from build123d import *

# Parameters (mm, degrees)
SKETCH10_W              = 71
SKETCH10_H              = 34
BOSS_EXTRUDE6_DEPTH     = 3.5
SKETCH11_R              = 1.55
CUT_EXTRUDE6_DEPTH      = 3.5
SKETCH12_R              = 2.75
CUT_EXTRUDE7_DEPTH      = 3.5
SKETCH13_R              = 3.75
BOSS_EXTRUDE7_DEPTH     = 25
CUT_EXTRUDE8_DEPTH      = 108.597630085
CUT_EXTRUDE8_DEPTH_BACK = 108.597630085
SKETCH14_R              = 1.55
FILLET6_R               = 8
FILLET7_R               = 8
SKETCH16_W              = 3
SKETCH16_H              = 4
SKETCH16_W_2            = 3.05572809
BOSS_EXTRUDE10_DEPTH    = 15
SKETCH18_W              = 3.05572809
SKETCH18_H              = 4.5
BOSS_EXTRUDE11_DEPTH    = 34


with BuildPart() as part:
    # Sketch10 → Boss-Extrude6 (new body)
    with BuildSketch(Plane(origin=(0, 0, 0), x_dir=(1, 0, 0), z_dir=(0, 1, 0))):
        with BuildLine():
            Line((0, -4), (0, -38))
            ThreePointArc((0, -38), (-0.190260598, -38.004527449), (-0.380090498, -38.018099548))
            Line((-0.380090498, -38.018099548), (-10.5, -38.5))
            ThreePointArc((-10.5, -38.5), (-14, -42), (-10.5, -45.5))
            Line((-10.5, -45.5), (-0.380090498, -45.981900452))
            ThreePointArc((-0.380090498, -45.981900452), (2.690691176, -44.959760294), (4, -42))
            Line((4, -42), (75, -42))
            ThreePointArc((75, -42), (76.309308824, -44.959760294), (79.380090498, -45.981900452))
            Line((79.380090498, -45.981900452), (89.5, -45.5))
            ThreePointArc((89.5, -45.5), (93, -42), (89.5, -38.5))
            Line((89.5, -38.5), (79.380090498, -38.018099548))
            ThreePointArc((79.380090498, -38.018099548), (79.190260598, -38.004527449), (79, -38))
            Line((79, -38), (79, -4))
            Line((79, -4), (89.5, -3.5))
            ThreePointArc((89.5, -3.5), (93, 0), (89.5, 3.5))
            Line((89.5, 3.5), (79, 4))
            ThreePointArc((79, 4), (76.171572875, 2.828427125), (75, 0))
            Line((75, 0), (4, 0))
            ThreePointArc((4, 0), (2.828427125, 2.828427125), (0, 4))
            Line((0, 4), (-10.5, 3.5))
            ThreePointArc((-10.5, 3.5), (-14, 0), (-10.5, -3.5))
            Line((-10.5, -3.5), (0, -4))
        make_face()
        with Locations((39.5, -21)):
            Rectangle(SKETCH10_W, SKETCH10_H, mode=Mode.SUBTRACT)
    extrude(amount=BOSS_EXTRUDE6_DEPTH)

    # Sketch11 → Cut-Extrude6 (cut)
    with BuildSketch(Plane(origin=(0, 3.5, 0), x_dir=(1, 0, 0), z_dir=(0, 1, 0))):
        with Locations(Location((0, 0, 0), (0, 0, 270))):
            Circle(SKETCH11_R)
        with Locations(Location((79, 0, 0), (0, 0, 270))):
            Circle(SKETCH11_R)
        with Locations(Location((79, -42, 0), (0, 0, 270))):
            Circle(SKETCH11_R)
        with Locations(Location((0, -42, 0), (0, 0, 270))):
            Circle(SKETCH11_R)
        with Locations(Location((-10.5, -42, 0), (0, 0, 270))):
            Circle(SKETCH11_R)
        with Locations(Location((-10.5, 0, 0), (0, 0, 270))):
            Circle(SKETCH11_R)
        with Locations(Location((89.5, 0, 0), (0, 0, 270))):
            Circle(SKETCH11_R)
        with Locations(Location((89.5, -42, 0), (0, 0, 270))):
            Circle(SKETCH11_R)
    extrude(amount=-CUT_EXTRUDE6_DEPTH, mode=Mode.SUBTRACT)

    # Sketch12 → Cut-Extrude7 (cut)
    with BuildSketch(Plane.XZ):
        with Locations(Location((0, 42, 0), (0, 0, 270))):
            Circle(SKETCH12_R)
        with Locations(Location((79, 42, 0), (0, 0, 270))):
            Circle(SKETCH12_R)
        with Locations(Location((79, 0, 0), (0, 0, 270))):
            Circle(SKETCH12_R)
        with Locations(Location((0, 0, 0), (0, 0, 270))):
            Circle(SKETCH12_R)
    extrude(amount=-CUT_EXTRUDE7_DEPTH, mode=Mode.SUBTRACT)

    # Sketch13 → Boss-Extrude7 (add)
    with BuildSketch(Plane(origin=(0, 3.5, 0), x_dir=(1, 0, 0), z_dir=(0, 1, 0))):
        with Locations(Location((0, 0, 0), (0, 0, 270))):
            Circle(SKETCH13_R)
        with Locations(Location((79, 0, 0), (0, 0, 270))):
            Circle(SKETCH13_R)
        with Locations(Location((79, -42, 0), (0, 0, 270))):
            Circle(SKETCH13_R)
        with Locations(Location((0, -42, 0), (0, 0, 270))):
            Circle(SKETCH13_R)
    extrude(amount=BOSS_EXTRUDE7_DEPTH)

    # Sketch14 → Cut-Extrude8 (cut, two sides: drawn at the far end of the back side and taken through both)
    with BuildSketch(Plane(origin=(0, 28.5, 0), x_dir=(1, 0, 0), z_dir=(0, 1, 0)).offset(-CUT_EXTRUDE8_DEPTH_BACK)):
        with Locations(Location((0, 0, 0), (0, 0, 270))):
            Circle(SKETCH14_R)
        with Locations(Location((79, 0, 0), (0, 0, 270))):
            Circle(SKETCH14_R)
        with Locations(Location((79, -42, 0), (0, 0, 270))):
            Circle(SKETCH14_R)
        with Locations(Location((0, -42, 0), (0, 0, 270))):
            Circle(SKETCH14_R)
    extrude(amount=CUT_EXTRUDE8_DEPTH + CUT_EXTRUDE8_DEPTH_BACK, mode=Mode.SUBTRACT)

    # Fillet6
    fillet6_edges = [part.edges().sort_by_distance(p)[0] for p in [
        (75, 1.75, 0),
        (4, 1.75, 0),
        (4, 1.75, 42),
        (75, 1.75, 42),
        (79, 1.75, 38),
        (79, 1.75, 4),
        (0, 1.75, 38),
        (0, 1.75, 4),
    ]]
    fillet(fillet6_edges, radius=FILLET6_R)

    # Fillet7
    fillet7_edges = [part.edges().sort_by_distance(p)[0] for p in [
        (75, 1.75, 38),
        (4, 1.75, 38),
        (4, 1.75, 4),
        (75, 1.75, 4),
    ]]
    fillet(fillet7_edges, radius=FILLET7_R)

    # Sketch16 → Boss-Extrude10 (add)
    with BuildSketch(Plane(origin=(0, 3.5, 0), x_dir=(1, 0, 0), z_dir=(0, 1, 0))):
        with Locations((10.44427191, -40)):
            Rectangle(SKETCH16_W, SKETCH16_H)
        with Locations((10.472135955, -2)):
            Rectangle(SKETCH16_W_2, SKETCH16_H)
    extrude(amount=BOSS_EXTRUDE10_DEPTH)

    # Sketch18 → Boss-Extrude11 (add)
    with BuildSketch(Plane.XY.offset(4)):
        with Locations((10.472135955, 16.25)):
            Rectangle(SKETCH18_W, SKETCH18_H)
    extrude(amount=BOSS_EXTRUDE11_DEPTH)


solid = part.part
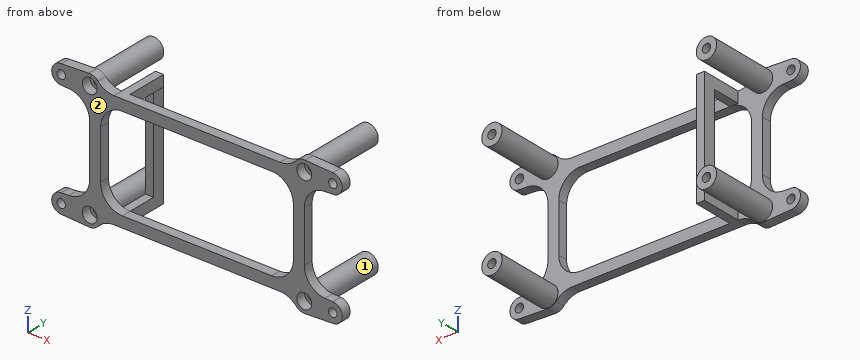
Can you work these out from the model? Positions are in its coordinate system, mm. Face numbers are marked on the shaded views. Coordinates: 2 decimals unless noted, no trailing zeros. Loops run counter-clockwise (first coordinate to the right, second up) from the corner with the lowest first, then second, coordinate; pieces in that order, holes last. Notation, with made-up numbers: M -12,59 L 24,59 A31 cw 24,97 Z; hole C 0,-7.5 d10. An arc over 180 degrees is marked long. Return JSON: item names as keys, results as strings. Group by question number.
Item 1: If I drill on L1, parallel to Z at x = 89.5, y = 2.65; L2, parallel to X at y = 2.5, z = 18; L3, parallel to Y at x = 56, z = 1, over which ranges is the centre line in solid material (lowest first)? Write a range as from..to.
Item 2: Imagine slicing it at A-A (y = 16). Give the number of separate pieces and of enclosed holes in the cut face, and give its area (3 significant figures).
Item 3: Imagine slicing it at B-B (z = 15.5). Please give me the cut outline in (x, y).
Item 4: Imagine slicing it at C-C (x = 61.5). Please give me the cut outline in (y, z).
Item 5: I'm going to push flat-ended pins straight in: pin 1 Ø1.6 at (x, z) = (78.5, 43) entering from -Y; pin 2 Ø2 at (x, z) = (10.5, 30.5) entering from -Y; pin 3 Ø1.5 at (x, z) = (42.5, 2) entering from +Y; pin 4 Ø8 at (x, y) = (61.5, 9.5) entering from +Z. Where does each tip first touch, or does it pass through?
Item 6: Thinking about a two-plate mould opening in X: for the marked faces 1 and 2, which applies, released by +X, released by -X, zero draft, split by the parting line, or undercut?
Verdict:
{
 "1": {"L1": "z = -3.5..-1.55, 1.55..3.5, 38.5..40.45, 43.55..45.5", "L2": "x = 0..4, 75..79", "L3": "y = 0..3.5"},
 "2": {"separate pieces": "5", "enclosed holes": "4", "area": "275 mm^2"},
 "3": {"outline": "M 0,0 L 4,0 L 4,3.5 L 0,3.5 Z; M 8.94,14 L 12,14 L 12,18.5 L 8.94,18.5 Z; M 75,0 L 79,0 L 79,3.5 L 75,3.5 Z"},
 "4": {"outline": "M 0,0 L 3.5,0 L 3.5,4 L 0,4 Z; M 0,38 L 3.5,38 L 3.5,42 L 0,42 Z"},
 "5": {"pin 1": "stops at y = 3.5", "pin 2": "stops at y = 14", "pin 3": "stops at y = 3.5", "pin 4": "passes through"},
 "6": {"face 1": "undercut", "face 2": "zero draft"}
}
